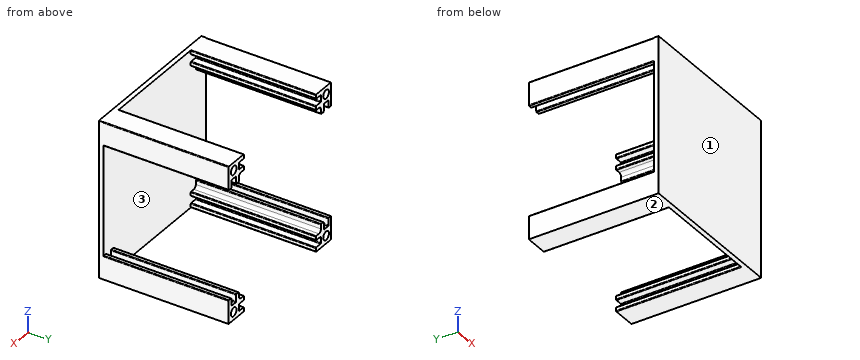
from build123d import *

# Parameters (mm, degrees)
SKETCH1_W           = 100
SKETCH1_H           = 100
BOSS_EXTRUDE1_DEPTH = 3
BOSS_EXTRUDE2_DEPTH = 80
SKETCH3_R           = 2.75
CUT_EXTRUDE1_DEPTH  = 6
FILLET3_R           = 2
FILLET4_R           = 0.5
MIRROR1_START       = 3
MIRROR1_DEPTH       = 74
MIRROR1_START_2     = 77
MIRROR1_2_OUTLINE_R = 2.75
MIRROR1_2_DEPTH     = 6


# Read off the part's stored shape, not the designer's step: Mirror1
with BuildPart() as part:
    # Sketch1 → Boss-Extrude1 (new body)
    with BuildSketch(Plane(origin=(0, 0, 0), x_dir=(1, 0, 0), z_dir=(0, 1, 0))):
        with Locations((50, 50)):
            Rectangle(SKETCH1_W, SKETCH1_H)
    extrude(amount=BOSS_EXTRUDE1_DEPTH)

    # Sketch2 → Boss-Extrude2 (add)
    with BuildSketch(Plane(origin=(0, 3, 0), x_dir=(1, 0, 0), z_dir=(0, 1, 0))):
        Polygon((0, 0), (10, 0), (15, 0), (15, 2.75), (10, 2.75), (10, 7.25), (15, 7.25), (15, 10), (10, 10), (10, 15), (7.25, 15), (7.25, 10), (2.75, 10), (2.75, 15), (0, 15), (0, 10), align=None)
    extrude(amount=BOSS_EXTRUDE2_DEPTH)

    # Sketch3 → Cut-Extrude1 (cut)
    with BuildSketch(Plane(origin=(0, 83, 0), x_dir=(1, 0, 0), z_dir=(0, 1, 0))):
        with Locations(Location((5, 5, 0), (0, 0, 270))):
            Circle(SKETCH3_R)
    extrude(amount=-CUT_EXTRUDE1_DEPTH, mode=Mode.SUBTRACT)

    # Fillet3
    fillet3_edges = [part.edges().sort_by_distance(p)[0] for p in [
        (10, 43, -10),
    ]]
    fillet(fillet3_edges, radius=FILLET3_R)

    # Fillet4
    fillet4_edges = [part.edges().sort_by_distance(p)[0] for p in [
        (7.25, 43, -10),
        (2.75, 43, -10),
        (10, 43, -7.25),
        (10, 43, -2.75),
        (0, 41.5, 0),
        (0, 43, -15),
        (2.75, 43, -15),
        (7.25, 43, -15),
        (10, 43, -15),
        (15, 43, -10),
        (15, 43, -7.25),
        (15, 43, -2.75),
        (15, 43, 0),
    ]]
    fillet(fillet4_edges, radius=FILLET4_R)

    # Mirror1 outline → Mirror1 (add)
    with BuildSketch(Plane(origin=(0, 0, 0), x_dir=(1, 0, 0), z_dir=(0, 1, 0)).offset(MIRROR1_START)):
        with BuildLine():
            Line((0, 100), (0, 85.5))
            ThreePointArc((0, 85.5), (0.146446609, 85.146446609), (0.5, 85))
            Line((0.5, 85), (2.25, 85))
            ThreePointArc((2.25, 85), (2.603553391, 85.146446609), (2.75, 85.5))
            Line((2.75, 85.5), (2.75, 89.5))
            ThreePointArc((2.75, 89.5), (2.896446609, 89.853553391), (3.25, 90))
            Line((3.25, 90), (6.75, 90))
            ThreePointArc((6.75, 90), (7.103553391, 89.853553391), (7.25, 89.5))
            Line((7.25, 89.5), (7.25, 85.5))
            ThreePointArc((7.25, 85.5), (7.396446609, 85.146446609), (7.75, 85))
            Line((7.75, 85), (9.5, 85))
            ThreePointArc((9.5, 85), (9.853553391, 85.146446609), (10, 85.5))
            Line((10, 85.5), (10, 88))
            ThreePointArc((10, 88), (10.585786438, 89.414213562), (12, 90))
            Line((12, 90), (14.5, 90))
            ThreePointArc((14.5, 90), (14.853553391, 90.146446609), (15, 90.5))
            Line((15, 90.5), (15, 92.25))
            ThreePointArc((15, 92.25), (14.853553391, 92.603553391), (14.5, 92.75))
            Line((14.5, 92.75), (10.5, 92.75))
            ThreePointArc((10.5, 92.75), (10.146446609, 92.896446609), (10, 93.25))
            Line((10, 93.25), (10, 96.75))
            ThreePointArc((10, 96.75), (10.146446609, 97.103553391), (10.5, 97.25))
            Line((10.5, 97.25), (14.5, 97.25))
            ThreePointArc((14.5, 97.25), (14.853553391, 97.396446609), (15, 97.75))
            Line((15, 97.75), (15, 99.5))
            ThreePointArc((15, 99.5), (14.853553391, 99.853553391), (14.5, 100))
            Line((14.5, 100), (0, 100))
        make_face()
    extrude(amount=MIRROR1_DEPTH)

    # Mirror1 2 outline → Mirror1 2 (add)
    with BuildSketch(Plane(origin=(0, 0, 0), x_dir=(1, 0, 0), z_dir=(0, 1, 0)).offset(MIRROR1_START_2)):
        with BuildLine():
            Line((0, 100), (0, 85.5))
            ThreePointArc((0, 85.5), (0.146446609, 85.146446609), (0.5, 85))
            Line((0.5, 85), (2.25, 85))
            ThreePointArc((2.25, 85), (2.603553391, 85.146446609), (2.75, 85.5))
            Line((2.75, 85.5), (2.75, 89.5))
            ThreePointArc((2.75, 89.5), (2.896446609, 89.853553391), (3.25, 90))
            Line((3.25, 90), (6.75, 90))
            ThreePointArc((6.75, 90), (7.103553391, 89.853553391), (7.25, 89.5))
            Line((7.25, 89.5), (7.25, 85.5))
            ThreePointArc((7.25, 85.5), (7.396446609, 85.146446609), (7.75, 85))
            Line((7.75, 85), (9.5, 85))
            ThreePointArc((9.5, 85), (9.853553391, 85.146446609), (10, 85.5))
            Line((10, 85.5), (10, 88))
            ThreePointArc((10, 88), (10.585786438, 89.414213562), (12, 90))
            Line((12, 90), (14.5, 90))
            ThreePointArc((14.5, 90), (14.853553391, 90.146446609), (15, 90.5))
            Line((15, 90.5), (15, 92.25))
            ThreePointArc((15, 92.25), (14.853553391, 92.603553391), (14.5, 92.75))
            Line((14.5, 92.75), (10.5, 92.75))
            ThreePointArc((10.5, 92.75), (10.146446609, 92.896446609), (10, 93.25))
            Line((10, 93.25), (10, 96.75))
            ThreePointArc((10, 96.75), (10.146446609, 97.103553391), (10.5, 97.25))
            Line((10.5, 97.25), (14.5, 97.25))
            ThreePointArc((14.5, 97.25), (14.853553391, 97.396446609), (15, 97.75))
            Line((15, 97.75), (15, 99.5))
            ThreePointArc((15, 99.5), (14.853553391, 99.853553391), (14.5, 100))
            Line((14.5, 100), (0, 100))
        make_face()
        with Locations((5, 95)):
            Circle(MIRROR1_2_OUTLINE_R, mode=Mode.SUBTRACT)
    extrude(amount=MIRROR1_2_DEPTH)

    # Mirror2: part across plane


with BuildPart() as part_1:
    add(part.part)
    add(part.part.mirror(Plane(origin=(50, 0, 0), x_dir=(0, 0, 1), z_dir=(1, 0, 0))))


solid = part_1.part
The listing builds one solid part. Answer for the finished solid, in the listing's coordinates (mm). Face numbers are marked on the shaded views. Give positions to 0.01 mm unless a question says otherwise; leave off trailing zeros. Write each loop counter-clockwise with the first axis right and the second up, starting at its lowest first coordinate (ties: lowest second). Pieces come first, ordered by that corner, then holes. Notation, with made-up numbers: (-35.5, 54) -> (-24.5, 54) arc R22 ccw to (-24.5, 88) -> close; hole circle Ø7 at (-36.75, -26.75). An arc over 180 degrees is marked (long way). One line per question, with ' | ' between items. Start each with the question number.
1. Given pin 1 Ø1.5 at (y, z) = (59, -17) entering from -X; pin 2 Ø10 at (x, z) = (81, -16) entering from +Y, each flat-ended and moving along its own axis, determine where each tip first touches the part or whether it passes through.
2. Section C-C (z = -95) is taken. Determine the outline of the cut face in (x, y), plus the area to 3 significant figures.
3. For a pull along Z with two mould halves and no side action, classify the marked faces 1, 2 and 3 as pulls with the +Z half, pulls with the -Z half, needs draft (parallel to the pull), parting line crosses it, or undercut.
4. Section A-A (x = 95) is taken. Determine the outline of the cut face in (y, z).
5. Section B-B (y = 60.5) is taken. State how many separate pieces and enclosed holes the cut face has, plus the area to 3 significant figures.
6. Find the intervals of material crossed by probe 1 along Z at (x, y) = (12.5, 42.5); probe 2 along Z at (x, y) = (95, 80.35); probe 3 along X at (y, z) = (79, -5), in increasing order.
7. Section D-D (z = -66) is taken. Determine the outline of the cut face in (x, y), plus the area to 3 significant figures.
Response values:
1) pin 1: through | pin 2: y = 3
2) outline: (0, 0) -> (100, 0) -> (100, 83) -> (97.75, 83) -> (97.75, 77) -> (92.25, 77) -> (92.25, 83) -> (90, 83) -> (90, 3) -> (10, 3) -> (10, 83) -> (7.75, 83) -> (7.75, 77) -> (2.25, 77) -> (2.25, 83) -> (0, 83) -> close | area: 1,830 mm2
3) face 1: needs draft | face 2: pulls with the -Z half | face 3: undercut
4) outline: (0, -100) -> (83, -100) -> (83, -97.75) -> (77, -97.75) -> (77, -92.25) -> (83, -92.25) -> (83, -90) -> (3, -90) -> (3, -10) -> (83, -10) -> (83, -7.75) -> (77, -7.75) -> (77, -2.25) -> (83, -2.25) -> (83, 0) -> (0, 0) -> close
5) separate pieces: 4 | enclosed holes: 0 | area: 622 mm2
6) probe 1: -100 to -97.25, -92.75 to -90, -10 to -7.25, -2.75 to 0 | probe 2: -100 to -97.75, -92.25 to -90, -10 to -7.75, -2.25 to 0 | probe 3: 0 to 2.25, 7.75 to 10, 90 to 92.25, 97.75 to 100
7) outline: (0, 0) -> (100, 0) -> (100, 3) -> (0, 3) -> close | area: 300 mm2
